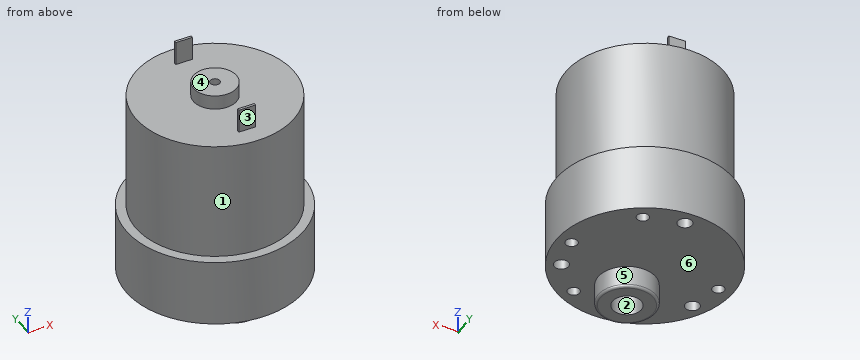
```python
from build123d import *

# Parameters (mm, degrees)
SKETCH1_R                 = 18.5
BOSS_EXTRUDE1_DEPTH       = 42
CUT_EXTRUDE1_START        = -3
SKETCH2_R                 = 18.5
SKETCH2_R_2               = 4.5
CUT_EXTRUDE1_DEPTH        = 3
CUT_EXTRUDE4_START        = -25
SKETCH3_R                 = 18.5
SKETCH3_R_2               = 16.5
CUT_EXTRUDE4_DEPTH        = 25
SKETCH4_R                 = 6
BOSS_EXTRUDE2_DEPTH       = 4.6
FILLET1_R                 = 0.5
SKETCH5_R                 = 3
CUT_EXTRUDE5_DEPTH        = 10
SKETCH6_R                 = 1
CUT_EXTRUDE6_DEPTH        = 10
SKETCH7_W                 = 3.5
SKETCH7_H                 = 0.5
BOSS_EXTRUDE3_DEPTH       = 5
M3X0_5_TAPPED_HOLE1_D     = 2.5
M3X0_5_TAPPED_HOLE1_DEPTH = 7.5
M3X0_5_TAPPED_HOLE1_TIP   = 0.751075774
F_3_0MM_DOWEL_HOLE1_D     = 3
F_3_0MM_DOWEL_HOLE1_DEPTH = 7.5
F_3_0MM_DOWEL_HOLE1_TIP   = 0.901290929


with BuildPart() as part:
    # Sketch1 → Boss-Extrude1 (new body)
    with BuildSketch(Plane.XY):
        with Locations(Location((0, 0, 0), (0, 0, 180))):
            Circle(SKETCH1_R)
    extrude(amount=BOSS_EXTRUDE1_DEPTH)

    # Sketch2 → Cut-Extrude1 (cut)
    with BuildSketch(Plane.XY.offset(42).offset(CUT_EXTRUDE1_START)):
        with Locations(Location((0, 0, 0), (0, 0, 180))):
            Circle(SKETCH2_R)
        Circle(SKETCH2_R_2, mode=Mode.SUBTRACT)
    extrude(amount=CUT_EXTRUDE1_DEPTH, mode=Mode.SUBTRACT)

    # Sketch3 → Cut-Extrude4 (cut)
    with BuildSketch(Plane.XY.offset(39).offset(CUT_EXTRUDE4_START)):
        with Locations(Location((0, 0, 0), (0, 0, 180))):
            Circle(SKETCH3_R)
        Circle(SKETCH3_R_2, mode=Mode.SUBTRACT)
    extrude(amount=CUT_EXTRUDE4_DEPTH, mode=Mode.SUBTRACT)

    # Sketch4 → Boss-Extrude2 (add)
    with BuildSketch(Plane(origin=(0, 0, 0), x_dir=(-1, 0, 0), z_dir=(0, 0, -1))):
        with Locations(Location((0, -7, 0), (0, 0, 180))):
            Circle(SKETCH4_R)
    extrude(amount=BOSS_EXTRUDE2_DEPTH)

    # Fillet1
    fillet1_edges = [part.edges().sort_by_distance(p)[0] for p in [
        (-6, -7, -4.6),
    ]]
    fillet(fillet1_edges, radius=FILLET1_R)

    # Sketch5 → Cut-Extrude5 (cut)
    with BuildSketch(Plane(origin=(0, 0, -4.6), x_dir=(-1, 0, 0), z_dir=(0, 0, -1))):
        with Locations((0, -7)):
            Circle(SKETCH5_R)
    extrude(amount=-CUT_EXTRUDE5_DEPTH, mode=Mode.SUBTRACT)

    # Sketch6 → Cut-Extrude6 (cut)
    with BuildSketch(Plane.XY.offset(42)):
        Circle(SKETCH6_R)
    extrude(amount=-CUT_EXTRUDE6_DEPTH, mode=Mode.SUBTRACT)

    # Sketch7 → Boss-Extrude3 (add)
    with BuildSketch(Plane.XY.offset(39)):
        with Locations((0, 12.25)):
            Rectangle(SKETCH7_W, SKETCH7_H)
        with Locations((0, -12.25)):
            Rectangle(SKETCH7_W, SKETCH7_H)
    extrude(amount=BOSS_EXTRUDE3_DEPTH)

    # M3x0.5 Tapped Hole1
    with Locations(Plane(origin=(0, 0, 0), x_dir=(-1, 0, 0), z_dir=(0, 0, -1))):
        with Locations((15.5, 0), (-7.75, 13.423393759), (-7.75, -13.423393759), (-15.5, 0)):
            Hole(M3X0_5_TAPPED_HOLE1_D / 2, depth=M3X0_5_TAPPED_HOLE1_DEPTH)
            with Locations((0, 0, -(M3X0_5_TAPPED_HOLE1_DEPTH + M3X0_5_TAPPED_HOLE1_TIP / 2))):  # 118° drill point
                Cone(0, M3X0_5_TAPPED_HOLE1_D / 2, M3X0_5_TAPPED_HOLE1_TIP, mode=Mode.SUBTRACT)

    # Ø3.0mm Dowel Hole1
    with Locations(Plane(origin=(0, 0, 0), x_dir=(-1, 0, 0), z_dir=(0, 0, -1))):
        with Locations((0, 15.5), (-13.829316686, -7), (13.829316686, -7)):
            Hole(F_3_0MM_DOWEL_HOLE1_D / 2, depth=F_3_0MM_DOWEL_HOLE1_DEPTH)
            with Locations((0, 0, -(F_3_0MM_DOWEL_HOLE1_DEPTH + F_3_0MM_DOWEL_HOLE1_TIP / 2))):  # 118° drill point
                Cone(0, F_3_0MM_DOWEL_HOLE1_D / 2, F_3_0MM_DOWEL_HOLE1_TIP, mode=Mode.SUBTRACT)


solid = part.part
```
Verification items for the finished model (mm, model axes). Face numbers are marked on the shaded views. A direction names the side the tool comes from. Give positions to 0.01 mm unless a question says otherwise; leave off trailing zeros. Order: outer loops, then holes, each group sorted by start corner. A loop starts at its lowest first (then second) coordinate and runs counter-clockwise, first axis right, second up. Notation, with made-up numbers: (-31, 3.5) -> (-25, 3.5) arc R22 ccw to (-25, 9.5) -> close; hole circle Ø6 at (-1, 40). An arc over 180 degrees is marked (long way). One line per item, written item: value.
(1) Scan lines: line 1 along Y through (x, z) = (0, 1.25); line 2 along Y through (x, z) = (0, -0.5); line 3 along Y through (x, z) = (-15, 3). Record each from-to range of solid material in increasing order. Write a range as [from, to].
Final values:
line 1: [-18.5, -10], [-4, 14], [17, 18.5]
line 2: [-13, -10], [-4, -1]
line 3: [-10.83, -7.94], [-6.06, -1.15], [1.15, 10.83]
(2) Sectioned sample at D-D on z = 30. Record the cut outline in (x, y).
Final values:
outline: circle Ø33 at (0, 0)
(3) Sectioned sample at B-B on x = -9. Record the cut outline in (y, z).
Final values:
outline: (-16.16, 0) -> (16.16, 0) -> (16.16, 14) -> (13.83, 14) -> (13.83, 39) -> (-13.83, 39) -> (-13.83, 14) -> (-16.16, 14) -> close
(4) Draft check along Y on the marked faces 4, 5 and 6. Enter one of: pulls with the +Y half, pulls with the -Y half, needs draft (parallel to the pull), parting line crosses it, or undercut.
Final values:
face 4: undercut
face 5: parting line crosses it
face 6: needs draft
(5) Sectioned sample at A-A on z = 40. Record the cut outline in (x, y).
Final values:
outline: circle Ø9 at (0, 0); (-1.75, -12.5) -> (1.75, -12.5) -> (1.75, -12) -> (-1.75, -12) -> close; (-1.75, 12) -> (1.75, 12) -> (1.75, 12.5) -> (-1.75, 12.5) -> close; hole circle Ø2 at (0, 0)
(6) Sectioned sample at C-C on y = 2.5. Record the cut outline in (x, z), then the cut area to 3 significant figures.
Final values:
outline: (-18.33, 0) -> (18.33, 0) -> (18.33, 14) -> (16.31, 14) -> (16.31, 39) -> (3.74, 39) -> (3.74, 42) -> (-3.74, 42) -> (-3.74, 39) -> (-16.31, 39) -> (-16.31, 14) -> (-18.33, 14) -> close
area: 1,350 mm^2
(7) Gauge pin test, flat ends, axial feed: pin 1 (4 mm diameter, centred on x = -13.83, y = -7, fed in from +Z); pin 2 (9.5 mm diameter, centred on x = 0, y = -7, fed in from +Z); pin 3 (4 mm diameter, centred on x = -12, z = 18.5, fed in from -Y). Record the tip position at first contact, or that the pin passes through.
Final values:
pin 1: z = 39
pin 2: z = 42
pin 3: y = -13.12
(8) Tool access check on the marked faces 1, 2 and 3. Record the directions out of +Z, -Z, +X, -X, +Y, -Y that give a thin tool (end or side, any length) a straight path to the whole face; none if there is none.
Final values:
face 1: +Z
face 2: -Z
face 3: +Z, +X, -X, -Y
